from build123d import *

# Parameters (mm, degrees)
SKETCH1_R           = 1
BOSS_EXTRUDE1_DEPTH = 4.2
SKETCH2_R           = 1.1
BOSS_EXTRUDE2_DEPTH = 4
SKETCH3_W           = 25
SKETCH3_H           = 4.2
BOSS_EXTRUDE3_DEPTH = 2
SKETCH4_W           = 25
SKETCH4_H           = 2
BOSS_EXTRUDE4_DEPTH = 0.6
BOSS_EXTRUDE5_START = -5.4
SKETCH1_3_R         = 1
BOSS_EXTRUDE5_DEPTH = 5.4
SKETCH4_2_W         = 25
SKETCH4_2_H         = 2
BOSS_EXTRUDE6_DEPTH = 5.4
CUT_EXTRUDE2_REACH  = 38.502
SKETCH5_W           = 25
SKETCH5_H           = 1.2
SKETCH6_W           = 2.096367106
SKETCH6_H           = 4.2
BOSS_EXTRUDE8_DEPTH = 21.5
SKETCH5_2_W         = 25
SKETCH5_2_H         = 1.2
CUT_EXTRUDE4_DEPTH  = 2.5


with BuildPart() as part:
    # Sketch1 → Boss-Extrude1 (new body)
    with BuildSketch(Plane(origin=(0, 0, 0), x_dir=(1, 0, 0), z_dir=(0, 1, 0))):
        Polygon((0, 0), (25, 0), (25, 24), (20.75, 24), (20.75, 2.5), (4.25, 2.5), (4.25, 24), (0, 24), align=None)
        with Locations(Location((2, 14.5, 0), (0, 0, 270))):
            Circle(SKETCH1_R, mode=Mode.SUBTRACT)
        with Locations(Location((2, 2, 0), (0, 0, 270))):
            Circle(SKETCH1_R, mode=Mode.SUBTRACT)
        with Locations(Location((23, 2, 0), (0, 0, 90))):
            Circle(SKETCH1_R, mode=Mode.SUBTRACT)
        with Locations(Location((23, 14.5, 0), (0, 0, 90))):
            Circle(SKETCH1_R, mode=Mode.SUBTRACT)
    extrude(amount=BOSS_EXTRUDE1_DEPTH)

    # Sketch2 → Boss-Extrude2 (add)
    with BuildSketch(Plane.ZY):
        with Locations((-14, 2.2)):
            Circle(SKETCH2_R)
    boss_extrude2 = extrude(amount=BOSS_EXTRUDE2_DEPTH)

    # Mirror1: Boss-Extrude2 across plane
    add(boss_extrude2.mirror(Plane.ZY.offset(-12.5)))

    # Sketch3 → Boss-Extrude3 (add)
    with BuildSketch(Plane.XY):
        with Locations((12.5, 2.1)):
            Rectangle(SKETCH3_W, SKETCH3_H)
    extrude(amount=BOSS_EXTRUDE3_DEPTH)

    # Sketch4 → Boss-Extrude4 (add)
    with BuildSketch(Plane.XZ):
        with Locations((12.5, 1)):
            Rectangle(SKETCH4_W, SKETCH4_H)
    extrude(amount=BOSS_EXTRUDE4_DEPTH)

    # Sketch1<3> → Boss-Extrude5 (add)
    with BuildSketch(Plane(origin=(0, 0, 0), x_dir=(1, 0, 0), z_dir=(0, 1, 0)).offset(BOSS_EXTRUDE5_START)):
        Polygon((0, 0), (25, 0), (25, 24), (20.75, 24), (20.75, 2.5), (4.25, 2.5), (4.25, 24), (0, 24), align=None)
        with Locations(Location((2, 14.5, 0), (0, 0, 270))):
            Circle(SKETCH1_3_R, mode=Mode.SUBTRACT)
        with Locations(Location((2, 2, 0), (0, 0, 270))):
            Circle(SKETCH1_3_R, mode=Mode.SUBTRACT)
        with Locations(Location((23, 2, 0), (0, 0, 90))):
            Circle(SKETCH1_3_R, mode=Mode.SUBTRACT)
        with Locations(Location((23, 14.5, 0), (0, 0, 90))):
            Circle(SKETCH1_3_R, mode=Mode.SUBTRACT)
    extrude(amount=BOSS_EXTRUDE5_DEPTH)

    # Sketch4<2> → Boss-Extrude6 (add)
    with BuildSketch(Plane.XZ):
        with Locations((12.5, 1)):
            Rectangle(SKETCH4_2_W, SKETCH4_2_H)
    extrude(amount=BOSS_EXTRUDE6_DEPTH)

    # Cut-Extrude2: up to this face of the body (flat: up to its plane)
    cut_extrude2_end = Plane(part.part.faces().sort_by_distance((22.875, -0.6, -24))[0])
    # Sketch5 → Cut-Extrude2 (cut, up to the picked face)
    with BuildSketch(Plane(origin=(0, 0, -2.5), x_dir=(-1, 0, 0), z_dir=(0, 0, -1)), mode=Mode.PRIVATE) as cut_extrude2_sk1:
        with Locations((-12.5, -0.6)):
            Rectangle(SKETCH5_W, SKETCH5_H)
    cut_extrude2_tool1 = split(extrude(cut_extrude2_sk1.sketch, amount=CUT_EXTRUDE2_REACH, mode=Mode.PRIVATE), bisect_by=cut_extrude2_end, keep=Keep.BOTH, mode=Mode.PRIVATE)
    add(cut_extrude2_tool1.solids().sort_by(Axis((12.5, -0.6, -2.5), (0, 0, -1)))[0], mode=Mode.SUBTRACT)

    # Sketch6 → Boss-Extrude8 (add)
    with BuildSketch(Plane(origin=(0, 0, -2.5), x_dir=(-1, 0, 0), z_dir=(0, 0, -1))):
        with Locations((-19.701816447, 2.1)):
            Rectangle(SKETCH6_W, SKETCH6_H)
        with Locations((-5.298183553, 2.1)):
            Rectangle(SKETCH6_W, SKETCH6_H)
        with Locations((-5.298183553, -3.3)):
            Rectangle(SKETCH6_W, SKETCH6_H)
        with Locations((-19.701816447, -3.3)):
            Rectangle(SKETCH6_W, SKETCH6_H)
    extrude(amount=BOSS_EXTRUDE8_DEPTH)

    # Sketch5<2> → Cut-Extrude4 (cut)
    with BuildSketch(Plane(origin=(0, 0, -2.5), x_dir=(-1, 0, 0), z_dir=(0, 0, -1))):
        with Locations((-12.5, -0.6)):
            Rectangle(SKETCH5_2_W, SKETCH5_2_H)
    extrude(amount=-CUT_EXTRUDE4_DEPTH, mode=Mode.SUBTRACT)


solid = part.part
Geometry: final body of the model. Coordinates: model frame, mm. A direction names the side the tool comes from. Coordinates: 2 decimals unless noted, no trailing zeros. Order: outer loops, then holes, each group sorted by start corner. A loop starts at its lowest first (then second) coordinate and runs counter-clockwise, first axis right, second up.
1) Section B-B (z = -2). Return loops of the section in (x, y), then the cut area to 3 significant figures.
Result sheet:
outline: (0, -5.4) - (1, -5.4) - (1, -1.2) - (0, -1.2) - close; (0, 0) - (1, 0) - (1, 4.2) - (0, 4.2) - close; (3, -5.4) - (22, -5.4) - (22, -1.2) - (3, -1.2) - close; (3, 0) - (22, 0) - (22, 4.2) - (3, 4.2) - close; (24, -5.4) - (25, -5.4) - (25, -1.2) - (24, -1.2) - close; (24, 0) - (25, 0) - (25, 4.2) - (24, 4.2) - close
area: 176 mm2
2) Section C-C (y = -4.5). Return loops of the section in (x, z).
Result sheet:
outline: (0, -24) - (6.35, -24) - (6.35, -2.5) - (18.65, -2.5) - (18.65, -24) - (25, -24) - (25, 2) - (0, 2) - close; hole circle Ø2 at (2, -14.5); hole circle Ø2 at (2, -2); hole circle Ø2 at (23, -14.5); hole circle Ø2 at (23, -2)
3) Ray query, probe 1 along Z at (x, y) = (2, -3.5); probe 2 along X at (y, z) = (1.55, -14.5); probe 3 along X at (y, z) = (-2.35, -14.5). Return the intervals inside material, ascending.
Result sheet:
probe 1: z = -24 to -15.5, -13.5 to -3, -1 to 2
probe 2: x = -4 to 1, 3 to 6.35, 18.65 to 22, 24 to 29
probe 3: x = 0 to 1, 3 to 6.35, 18.65 to 22, 24 to 25
4) Set-up query: faces 1 (the cylindrical face through (23.89, -3.33, -14.96)), 2 (the flat face through (21, 0, -12)), 3 (the flat face through (13, -3, -2.5)). Return all of +Z, -Z, +X, -X, +Y, -Y with unobstructed straight access to the full face (end or side cutting, diameter ignored); none if empty.
Result sheet:
face 1: +Y, -Y
face 2: -Z, +X, -X
face 3: -Z, +Y, -Y
5) Section A-A (x = 23). Return loops of the section in (y, z), then the cut area to 3 significant figures.
Result sheet:
outline: (-5.4, -24) - (-1.2, -24) - (-1.2, -15.5) - (-5.4, -15.5) - close; (-5.4, -13.5) - (-1.2, -13.5) - (-1.2, -3) - (-5.4, -3) - close; (-5.4, -1) - (-1.2, -1) - (-1.2, 0) - (0, 0) - (0, -1) - (4.2, -1) - (4.2, 2) - (-5.4, 2) - close; (0, -24) - (4.2, -24) - (4.2, -15.5) - (0, -15.5) - close; (0, -13.5) - (4.2, -13.5) - (4.2, -3) - (0, -3) - close
area: 187 mm2
6) First-contact query: P1, Ø1, axis at y = -2, z = -2.5, coming from the -X side; P2, Ø1.2, axis at x = 23, z = -14.5, coming from the +Y side; P3, Ø3.5, axis at x = 15.5, y = 2.5, coming from the -Z side; P4, Ø2, axis at y = -3, z = -10.5, coming from the +X side. Flat tips, straight axial feed; report the tip coordinate or a pass-through.
Result sheet:
P1: stops at x = 0
P2: passes through
P3: stops at z = -2.5
P4: stops at x = 25
7) Section D-D (z = -10). Return loops of the section in (x, y), then the cut area to 3 significant figures.
Result sheet:
outline: (0, -5.4) - (6.35, -5.4) - (6.35, -1.2) - (0, -1.2) - close; (0, 0) - (6.35, 0) - (6.35, 4.2) - (0, 4.2) - close; (18.65, -5.4) - (25, -5.4) - (25, -1.2) - (18.65, -1.2) - close; (18.65, 0) - (25, 0) - (25, 4.2) - (18.65, 4.2) - close
area: 107 mm2
8) Draft query along Z for faces 4 (the flat face through (22, 2, -24)), 5 (the flat face through (18.654, 2, -13)), 6 (the cylindrical face through (1.4, 2.1, -2.8)). Return one class per face: released by +Z, released by -Z, zero draft, split by the parting line, or undercut.
Result sheet:
face 4: released by -Z
face 5: zero draft
face 6: undercut
